Read the model definition and answer for the solid it produces. Units are mm, in the model's axes. A direction names the side the tool comes from. Give positions to 0.01 mm unless a question says otherwise; leave off trailing zeros. Write each loop counter-clockwise with the first axis right and the second up, starting at its lowest first coordinate (ties: lowest second). Pieces come first, ordered by that corner, then holes. Notation, with made-up numbers: (58.25, 54) - (76.25, 54) arc R12 ccw to (76.25, 60) - close; hole circle Ø7 at (65.25, 64.5). An arc over 180 degrees is marked (long way). Answer as CSV lines item,"result".
```python
from build123d import *

# Parameters (mm, degrees)
SKETCH1_W           = 144.78
SKETCH1_H           = 38.1
SKETCH1_R           = 1.7
BOSS_EXTRUDE1_DEPTH = 12.7
SKETCH2_R           = 6.6
CUT_EXTRUDE1_DEPTH  = 5.08
SKETCH4_R           = 6.35
SKETCH4_R_2         = 1.7
BOSS_EXTRUDE2_DEPTH = 38.1
FILLET1_R           = 1.27
CHAMFER1_SIZE       = 0.5


with BuildPart() as part:
    # Sketch1 → Boss-Extrude1 (new body)
    with BuildSketch(Plane(origin=(0, 0, 0), x_dir=(1, 0, 0), z_dir=(0, 1, 0))):
        with Locations((72.39, 19.05)):
            Rectangle(SKETCH1_W, SKETCH1_H)
        with Locations(Location((59.69, 19.05, 0), (0, 0, 270))):
            Circle(SKETCH1_R, mode=Mode.SUBTRACT)
        with Locations(Location((85.09, 19.05, 0), (0, 0, 270))):
            Circle(SKETCH1_R, mode=Mode.SUBTRACT)
    extrude(amount=BOSS_EXTRUDE1_DEPTH)

    # Sketch2 → Cut-Extrude1 (cut)
    with BuildSketch(Plane(origin=(0, 12.7, 0), x_dir=(1, 0, 0), z_dir=(0, 1, 0))):
        with Locations(Location((24.765, 19.05, 0), (0, 0, 270))):
            Circle(SKETCH2_R)
        with Locations(Location((120.015, 19.05, 0), (0, 0, 90))):
            Circle(SKETCH2_R)
    extrude(amount=-CUT_EXTRUDE1_DEPTH, mode=Mode.SUBTRACT)

    # Sketch4 → Boss-Extrude2 (add)
    # profile 1 of 4: a face of its own
    with BuildSketch(Plane(origin=(0, 12.7, 0), x_dir=(1, 0, 0), z_dir=(0, 1, 0))):
        with Locations(Location((85.09, 19.05, 0), (0, 0, 90))):
            Circle(SKETCH4_R)
        with Locations(Location((85.09, 19.05, 0), (0, 0, 270))):
            Circle(SKETCH4_R_2, mode=Mode.SUBTRACT)
    # profile 2 of 4: a face of its own
    with BuildSketch(Plane(origin=(0, 12.7, 0), x_dir=(1, 0, 0), z_dir=(0, 1, 0))):
        with Locations(Location((59.69, 19.05, 0), (0, 0, 90))):
            Circle(SKETCH4_R)
        with Locations(Location((59.69, 19.05, 0), (0, 0, 270))):
            Circle(SKETCH4_R_2, mode=Mode.SUBTRACT)
    # profile 3 of 4: a face of its own
    with BuildSketch(Plane(origin=(0, 12.7, 0), x_dir=(1, 0, 0), z_dir=(0, 1, 0))):
        with BuildLine():
            Line((24.765, 33.02), (24.765, 29.21))
            ThreePointArc((24.765, 29.21), (14.605, 19.05), (24.765, 8.89))
            Line((24.765, 8.89), (24.765, 5.08))
            ThreePointArc((24.765, 5.08), (10.795, 19.05), (24.765, 33.02))
        make_face()
    # profile 4 of 4: a face of its own
    with BuildSketch(Plane(origin=(0, 12.7, 0), x_dir=(1, 0, 0), z_dir=(0, 1, 0))):
        with BuildLine():
            Line((120.015, 8.89), (120.015, 5.08))
            ThreePointArc((120.015, 5.08), (133.985, 19.05), (120.015, 33.02))
            Line((120.015, 33.02), (120.015, 29.21))
            ThreePointArc((120.015, 29.21), (130.175, 19.05), (120.015, 8.89))
        make_face()
    extrude(amount=BOSS_EXTRUDE2_DEPTH)

    # Fillet1
    fillet1_edges = [part.edges().sort_by_distance(p)[0] for p in [
        (85.09, 12.7, -12.7),
        (59.69, 12.7, -12.7),
        (14.605, 12.7, -19.05),
        (24.765, 12.7, -31.115),
        (10.795, 12.7, -19.05),
        (24.765, 12.7, -6.985),
        (130.175, 12.7, -19.05),
        (120.015, 12.7, -6.985),
        (133.985, 12.7, -19.05),
        (120.015, 12.7, -31.115),
    ]]
    fillet(fillet1_edges, radius=FILLET1_R)

    # Chamfer1
    chamfer1_edges = [part.edges().sort_by_distance(p)[0] for p in [
        (59.69, 0, -20.75),
        (85.09, 0, -20.75),
        (72.39, 0, -38.1),
        (144.78, 0, -19.05),
        (72.39, 0, 0),
        (0, 0, -19.05),
    ]]
    chamfer(chamfer1_edges, length=CHAMFER1_SIZE)


solid = part.part
```
(1) A cutting plane is placed at B-B (x = 85.09). Write down the section's boundary in (y, z).
Worked out:
outline,"(0, -37.6) - (0.5, -38.1) - (12.7, -38.1) - (12.7, -26.67) arc R1.27 cw to (13.97, -25.4) - (50.8, -25.4) - (50.8, -20.75) - (0.5, -20.75) - (0, -21.25) - close; (0, -16.85) - (0.5, -17.35) - (50.8, -17.35) - (50.8, -12.7) - (13.97, -12.7) arc R1.27 cw to (12.7, -11.43) - (12.7, 0) - (0.5, 0) - (0, -0.5) - close"
(2) A cutting plane is placed at A-A (y = 21.5). Write down the section's boundary in (x, z) (3 decimals).
Worked out:
outline,"(24.765, -33.02) - (24.765, -29.21) arc R10.16 cw to (24.765, -8.89) - (24.765, -5.08) arc R13.97 ccw to start; circle Ø12.7 at (59.69, -19.05); circle Ø12.7 at (85.09, -19.05); (120.015, -33.02) arc R13.97 ccw to (120.015, -5.08) - (120.015, -8.89) arc R10.16 cw to (120.015, -29.21) - close; hole circle Ø3.4 at (59.69, -19.05); hole circle Ø3.4 at (85.09, -19.05)"
(3) The mould has two halves that part along X. Classify faces 1 (the flat face through (120.015, 32, -7)), 2 (the flat face through (130, 50.8, -22)), 3 (the cylindrical face through (22.24, 10.2, -12.95)), 4 (the flat face through (0, 7, -19)): +X half, -X half, draft (parallel to the pull), parting line (faces both ways), or undercut.
Worked out:
face 1,"undercut"
face 2,"draft"
face 3,"undercut"
face 4,"-X half"
(4) Each of these flat-tipped pins is pushed along its axis until it touches: P1, Ø4, axis at x = 23, y = 17.5, coming from the +Z side; P2, Ø1.1, axis at y = 38.5, z = -31, coming from the -X side; P3, Ø12, axis at x = 32, z = -19, coming from the +Y side; P4, Ø3, axis at x = 85.09, z = -19.05, coming from the +Y side. Where does it stop, or does it pass through?
Worked out:
P1,"stops at z = -5.08"
P2,"stops at x = 16.69"
P3,"stops at y = 12.7"
P4,"passes through"
(5) A cutting plane is placed at D-D (z = -19.05). Count the separate pieces of the cut face and the enclosed holes in it, and give its area (3 significant figures).
Worked out:
separate pieces,"3"
enclosed holes,"0"
area,"2,620 mm^2"
(6) For faces 5 (the cylindrical face through (130.173, 32.127, -19.273)), 6 (the cylindrical face through (133.98, 32.13, -18.74)), 7 (the flat face through (24.765, 32, -31)), determine the directions among +Z, -Z, +X, -X, +Y, -Y from which every point of the face is accessible in a straight line to the end or side of a thin tool.
Worked out:
face 5,"+Y"
face 6,"+X, +Y"
face 7,"+Z, -Z, +Y"
(7) A cutting plane is placed at C-C (x = 70.5). Write down the section's boundary in (y, z).
Worked out:
outline,"(0, -37.6) - (0.5, -38.1) - (12.7, -38.1) - (12.7, 0) - (0.5, 0) - (0, -0.5) - close"
(8) Find the intervals of material crossed by L1, parallel to X at y = 10, z = -19; L2, parallel to X at y = 32.5, z = -19.05 (3 decimals); L3, parallel to Z at x = 85, y = 42, in increasing order.
Worked out:
L1,"x = 0 to 18.17, 31.36 to 57.99, 61.39 to 83.39, 86.79 to 113.42, 126.61 to 144.78"
L2,"x = 10.795 to 14.605, 53.34 to 57.99, 61.39 to 66.04, 78.74 to 83.39, 86.79 to 91.44, 130.175 to 133.985"
L3,"z = -25.4 to -20.75, -17.35 to -12.7"
